Can you work these out from the model? Positions are in its coordinate system, mm. Face numbers are marked on the shaded views. A direction names the side the tool comes from. Round coordinates to 2 decimals unless told otherwise and drop trailing zeros. Loops run counter-clockwise (first coordinate to the right, second up) from the corner with the lowest first, then second, coordinate; pieces in that order, holes last.
(1) Will these pins go through, and if not, where does the flat tip stop? pin 1 Ø5 at (x, z) = (21, -21.5) entering from -Y; pin 2 Ø1.2 at (x, y) = (-1, -25) entering from -Z; pin 3 Ø12 at (y, z) = (-21.5, -22) entering from -X.
(2) I want a section at B-B on z = -5.5. Write out the boundary of the cut face in (x, y), plus the area to 3 significant figures.
(3) Which directions (+Z, -Z, +X, -X, +Y, -Y) give clear straight access to the entire face, cutting with the end or side of a thin tool? Please do the marked faces 1 and 2.
(4) If I drill on line 1 along X through (y, z) = (21, 17); line 2 along Z through (x, y) = (25.5, 19), over which ranges is the centre line in solid material (lowest first)?
(5) I want a section at A-A on y = 0. Write out the boundary of the cut face in (x, z) (3 decimals), plus the area to 3 significant figures.
from build123d import *

# Parameters (mm, degrees)
ESQUISSE1_W             = 55.5
ESQUISSE1_H             = 55.5
BOSS_EXTRU_1_DEPTH      = 19.5
ESQUISSE2_R             = 25
BOSS_EXTRU_2_DEPTH      = 18
ESQUISSE3_R             = 22.125
BOSS_EXTRU_3_DEPTH      = 13.5
CHANFREIN1_SIZE         = 3
CONG_1_R                = 1
CONG_2_R                = 10
ESQUISSE4_R             = 1.5
ENL_V_MAT_EXTRU_1_DEPTH = 4
ESQUISSE5_W             = 14.5
ESQUISSE5_H             = 2.5
ENL_V_MAT_EXTRU_2_DEPTH = 4


with BuildPart() as part:
    # Esquisse1 → Boss.-Extru.1 (new body)
    with BuildSketch(Plane.XY):
        Rectangle(ESQUISSE1_W, ESQUISSE1_H)
    extrude(amount=BOSS_EXTRU_1_DEPTH)

    # Esquisse2 → Boss.-Extru.2 (add)
    with BuildSketch(Plane(origin=(0, 0, 0), x_dir=(-1, 0, 0), z_dir=(0, 0, -1))):
        Circle(ESQUISSE2_R)
    extrude(amount=BOSS_EXTRU_2_DEPTH)

    # Esquisse3 → Boss.-Extru.3 (add)
    with BuildSketch(Plane(origin=(0, 0, -18), x_dir=(-1, 0, 0), z_dir=(0, 0, -1))):
        Circle(ESQUISSE3_R)
    extrude(amount=BOSS_EXTRU_3_DEPTH)

    # Chanfrein1
    chanfrein1_edges = [part.edges().sort_by_distance(p)[0] for p in [
        (22.125, 0, -31.5),
    ]]
    chamfer(chanfrein1_edges, length=CHANFREIN1_SIZE)

    # Congé1
    cong_1_edges = [part.edges().sort_by_distance(p)[0] for p in [
        (27.75, 0, 19.5),
        (25, 0, 0),
        (25, 0, -18),
        (0, 27.75, 19.5),
        (22.125, 0, -18),
        (-27.75, 0, 19.5),
        (0, 27.75, 0),
        (27.75, 0, 0),
        (0, -27.75, 0),
        (-27.75, 0, 0),
        (0, -27.75, 19.5),
    ]]
    fillet(cong_1_edges, radius=CONG_1_R)

    # Congé2
    # the kernel refuses this fillet: 10 mm, written as the material it takes off along each edge
    with BuildSketch(Plane(origin=(17.75, -17.75, 19.5), x_dir=(0, -1, 0), z_dir=(-1, 0, 0))) as cong_2_piece_1:
        with BuildLine():
            CenterArc((9, -1), 1, 0, 90)
            Line((10, -1), (10, 0))
            Line((10, 0), (9, 0))
        make_face()
    revolve(axis=Axis((17.75, -17.75, 19.5), (0, 0, 1)), revolution_arc=90, mode=Mode.SUBTRACT)
    with BuildSketch(Plane(origin=(-17.75, -17.75, 19.5), x_dir=(-1, 0, 0), z_dir=(0, 1, 0))) as cong_2_piece_2:
        with BuildLine():
            CenterArc((9, -1), 1, 0, 90)
            Line((10, -1), (10, 0))
            Line((10, 0), (9, 0))
        make_face()
    revolve(axis=Axis((-17.75, -17.75, 19.5), (0, 0, 1)), revolution_arc=90, mode=Mode.SUBTRACT)
    with BuildSketch(Plane(origin=(17.75, 17.75, 19.5), x_dir=(1, 0, 0), z_dir=(0, -1, 0))) as cong_2_piece_3:
        with BuildLine():
            CenterArc((9, -1), 1, 0, 90)
            Line((10, -1), (10, 0))
            Line((10, 0), (9, 0))
        make_face()
    revolve(axis=Axis((17.75, 17.75, 19.5), (0, 0, 1)), revolution_arc=90, mode=Mode.SUBTRACT)
    with BuildSketch(Plane(origin=(-17.75, 17.75, 19.5), x_dir=(0, 1, 0), z_dir=(1, 0, 0))) as cong_2_piece_4:
        with BuildLine():
            CenterArc((9, -1), 1, 0, 90)
            Line((10, -1), (10, 0))
            Line((10, 0), (9, 0))
        make_face()
    revolve(axis=Axis((-17.75, 17.75, 19.5), (0, 0, 1)), revolution_arc=90, mode=Mode.SUBTRACT)
    with BuildSketch(Plane(origin=(17.75, 17.75, 0), x_dir=(0, 1, 0), z_dir=(-1, 0, 0))) as cong_2_piece_5:
        with BuildLine():
            CenterArc((9, -1), 1, 0, 90)
            Line((10, -1), (10, 0))
            Line((10, 0), (9, 0))
        make_face()
    revolve(axis=Axis((17.75, 17.75, 0), (0, 0, -1)), revolution_arc=90, mode=Mode.SUBTRACT)
    with BuildSketch(Plane(origin=(17.75, -17.75, 0), x_dir=(1, 0, 0), z_dir=(0, 1, 0))) as cong_2_piece_6:
        with BuildLine():
            CenterArc((9, -1), 1, 0, 90)
            Line((10, -1), (10, 0))
            Line((10, 0), (9, 0))
        make_face()
    revolve(axis=Axis((17.75, -17.75, 0), (0, 0, -1)), revolution_arc=90, mode=Mode.SUBTRACT)
    with BuildSketch(Plane(origin=(-17.75, 17.75, 0), x_dir=(-1, 0, 0), z_dir=(0, -1, 0))) as cong_2_piece_7:
        with BuildLine():
            CenterArc((9, -1), 1, 0, 90)
            Line((10, -1), (10, 0))
            Line((10, 0), (9, 0))
        make_face()
    revolve(axis=Axis((-17.75, 17.75, 0), (0, 0, -1)), revolution_arc=90, mode=Mode.SUBTRACT)
    with BuildSketch(Plane(origin=(-17.75, -17.75, 0), x_dir=(0, -1, 0), z_dir=(1, 0, 0))) as cong_2_piece_8:
        with BuildLine():
            CenterArc((9, -1), 1, 0, 90)
            Line((10, -1), (10, 0))
            Line((10, 0), (9, 0))
        make_face()
    revolve(axis=Axis((-17.75, -17.75, 0), (0, 0, -1)), revolution_arc=90, mode=Mode.SUBTRACT)
    with BuildSketch(Plane(origin=(-27.75, 27.75, 0), x_dir=(1, 0, 0), z_dir=(0, 0, 1)), Plane(origin=(-27.75, -27.75, 0), x_dir=(0, 1, 0), z_dir=(0, 0, 1))) as cong_2_piece_9:
        with BuildLine():
            CenterArc((CONG_2_R, -CONG_2_R), CONG_2_R, 90, 90)
            Line((0, -CONG_2_R), (0, 0))
            Line((0, 0), (CONG_2_R, 0))
        make_face()
    extrude(amount=19.5, mode=Mode.SUBTRACT)
    with BuildSketch(Plane(origin=(27.75, 27.75, 0), x_dir=(-1, 0, 0), z_dir=(0, 0, 1)), Plane(origin=(27.75, -27.75, 0), x_dir=(0, 1, 0), z_dir=(0, 0, 1))) as cong_2_piece_10:
        with BuildLine():
            CenterArc((CONG_2_R, CONG_2_R), CONG_2_R, 180, 90)
            Line((0, CONG_2_R), (0, 0))
            Line((0, 0), (CONG_2_R, 0))
        make_face()
    extrude(amount=19.5, mode=Mode.SUBTRACT)

    # Esquisse4 → Enlèv. mat.-Extru.1 (cut)
    with BuildSketch(Plane.XY.offset(19.5)):
        with Locations((-21.75, 21.75)):
            Circle(ESQUISSE4_R)
        with Locations((21.75, 21.75)):
            Circle(ESQUISSE4_R)
        with Locations((21.75, -21.75)):
            Circle(ESQUISSE4_R)
        with Locations((-21.75, -21.75)):
            Circle(ESQUISSE4_R)
    extrude(amount=-ENL_V_MAT_EXTRU_1_DEPTH, mode=Mode.SUBTRACT)

    # Esquisse5 → Enlèv. mat.-Extru.2 (cut)
    with BuildSketch(Plane.XZ.offset(27.75)):
        with Locations((0, 15.25)):
            Rectangle(ESQUISSE5_W, ESQUISSE5_H)
    extrude(amount=-ENL_V_MAT_EXTRU_2_DEPTH, mode=Mode.SUBTRACT)


solid = part.part
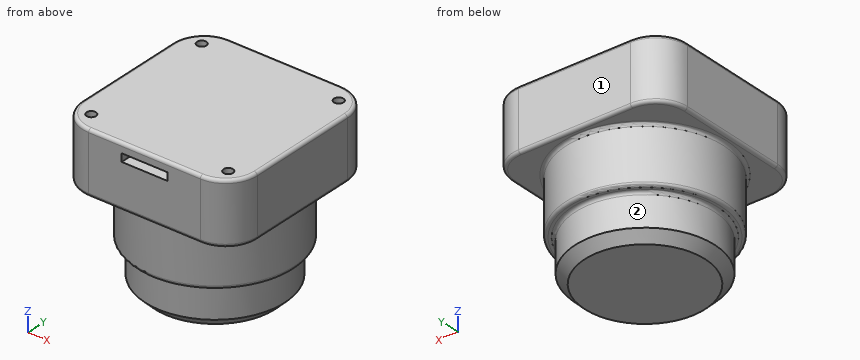
Filled sheet:
1. pin 1: stops at y = -12.14
1. pin 2: stops at z = -17.91
1. pin 3: stops at x = -17.65
2. outline: circle Ø50 at (0, 0)
2. area: 1,960 mm2
3. face 1: +Z, -Z, +X, -X, +Y
3. face 2: -Z
4. line 1: x = -27.21 to -23.05, -20.45 to 20.45, 23.05 to 27.21
4. line 2: z = 0 to 19.5
5. outline: (-27.75, 1) arc R1 ccw to (-26.75, 0) - (-26, 0) arc R1 cw to (-25, -1) - (-25, -17) arc R1 ccw to (-24, -18) - (-23.125, -18) arc R1 cw to (-22.125, -19) - (-22.125, -28.5) - (-19.125, -31.5) - (19.125, -31.5) - (22.125, -28.5) - (22.125, -19) arc R1 cw to (23.125, -18) - (24, -18) arc R1 ccw to (25, -17) - (25, -1) arc R1 cw to (26, 0) - (26.75, 0) arc R1 ccw to (27.75, 1) - (27.75, 18.5) arc R1 ccw to (26.75, 19.5) - (-26.75, 19.5) arc R1 ccw to (-27.75, 18.5) - close
5. area: 2,570 mm2
